Here's how the part is built. I have some questions about the finished solid (model axes, mm). A direction names the side the tool comes from. Give positions to 0.01 mm unless a question says otherwise; leave off trailing zeros. Write each loop counter-clockwise with the first axis right and the second up, starting at its lowest first coordinate (ties: lowest second). Pieces come first, ordered by that corner, then holes. Notation, with made-up numbers: (55, 51) -> (73, 51) arc R33 cw to (73, 82) -> close; hole circle Ø7 at (-17.75, 19). An arc over 180 degrees is marked (long way). Return JSON: item names as keys, results as strings.
from build123d import *

# Parameters (mm, degrees)
HOLE_WIZARD_M8_1_D           = 6.8
HOLE_WIZARD_M8_1_CSINK_D     = 8.05
HOLE_WIZARD_M8_1_CSINK_ANGLE = 90


with BuildPart() as part:
    # 草图1 → 旋转1 (revolve)
    with BuildSketch(Plane.XY, mode=Mode.PRIVATE) as revolve_1_sk:
        Polygon((0, 0), (77.5, 0), (77.5, 8), (45, 8), (45, 21), (37.5, 21), (37.5, 8), (0, 8), align=None)
    revolve(revolve_1_sk.sketch.rotate(Axis((0, 8, 0), (0, -1, 0)), 180), axis=Axis((0, 8, 0), (0, -1, 0)))

    # M8 螺纹孔1 (through all)
    with Locations(Plane(origin=(0, 8, 0), x_dir=(1, 0, 0), z_dir=(0, 1, 0))):
        with Locations((-67.5, 0), (67.5, 0), (0, -67.5), (0, 67.5)):
            CounterSinkHole(HOLE_WIZARD_M8_1_D / 2, HOLE_WIZARD_M8_1_CSINK_D / 2, counter_sink_angle=HOLE_WIZARD_M8_1_CSINK_ANGLE)


solid = part.part
1. Suppose I cut it at D-D, the plane x = 16. List the corners of the cut face in (y, z) for me, and give its area (3 significant figures).
Taken from the geometry:
{"outline": "(0, -75.83) -> (8, -75.83) -> (8, -42.06) -> (21, -42.06) -> (21, -33.92) -> (8, -33.92) -> (8, 33.92) -> (21, 33.92) -> (21, 42.06) -> (8, 42.06) -> (8, 75.83) -> (0, 75.83) -> close", "area": "1,430 mm²"}
2. Which directions (+Z, -Z, +X, -X, +Y, -Y) give clear straight access to the entire face, cutting with the end or side of a thin tool? Please do faces 1 (the face through (1, 8, -1)), 2 (the face through (17, 21, -34)).
Taken from the geometry:
{"face 1": "+Y", "face 2": "+Z, -Z, +X, -X, +Y"}
3. If I drill on line 1 (Z direction, x = 0, y = 4); line 2 (Y direction, x = -69, z = -4.5); line 3 (X direction, y = 4.5, z = 67.5), over which ranges is the centre line in solid material (lowest first)? Write a range as [from, to].
Taken from the geometry:
{"line 1": "z = [-77.5, -70.9], [-64.1, 64.1], [70.9, 77.5]", "line 2": "y = [0, 8]", "line 3": "x = [-38.08, -3.4], [3.4, 38.08]"}
4. For pin 1 Ø10 at (x, y) = (57, 2.5) entering from +Z; pin 2 Ø9 at (x, z) = (0, 67.5) entering from -Y; pin 3 Ø5 at (y, z) = (7, -56) entering from -X; pin 4 Ø1.5 at (x, y) = (3, 16) entering from -Z, each with a flat end and sliding along its axis, tell me the tip position at first contact or that it passes through.
Taken from the geometry:
{"pin 1": "stops at z = 57.47", "pin 2": "stops at y = 0", "pin 3": "stops at x = -56.07", "pin 4": "stops at z = -44.94"}
5. Suppose I cut it at C-C, the plane z = -67.5. List the corners of the cut face in (x, y) for me (3 decimals), and give its area (3 significant figures).
Taken from the geometry:
{"outline": "(-38.079, 0) -> (-3.4, 0) -> (-3.4, 7.375) -> (-4.025, 8) -> (-38.079, 8) -> close; (3.4, 0) -> (38.079, 0) -> (38.079, 8) -> (4.025, 8) -> (3.4, 7.375) -> close", "area": "554 mm²"}
6. Suppose I cut it at A-A, the plane z = 0. List the corners of the cut face in (x, y) for me (3 decimals), and give its area (3 significant figures).
Taken from the geometry:
{"outline": "(-77.5, 0) -> (-70.9, 0) -> (-70.9, 7.375) -> (-71.525, 8) -> (-77.5, 8) -> close; (-64.1, 0) -> (64.1, 0) -> (64.1, 7.375) -> (63.475, 8) -> (45, 8) -> (45, 21) -> (37.5, 21) -> (37.5, 8) -> (-37.5, 8) -> (-37.5, 21) -> (-45, 21) -> (-45, 8) -> (-63.475, 8) -> (-64.1, 7.375) -> close; (70.9, 0) -> (77.5, 0) -> (77.5, 8) -> (71.525, 8) -> (70.9, 7.375) -> close", "area": "1,330 mm²"}
7. Suppose I cut it at B-B, the plane x = 0. List the corners of the cut face in (y, z) for me (3 decimals).
Taken from the geometry:
{"outline": "(0, -77.5) -> (8, -77.5) -> (8, -71.525) -> (7.375, -70.9) -> (0, -70.9) -> close; (0, -64.1) -> (7.375, -64.1) -> (8, -63.475) -> (8, -45) -> (21, -45) -> (21, -37.5) -> (8, -37.5) -> (8, 37.5) -> (21, 37.5) -> (21, 45) -> (8, 45) -> (8, 63.475) -> (7.375, 64.1) -> (0, 64.1) -> close; (0, 70.9) -> (7.375, 70.9) -> (8, 71.525) -> (8, 77.5) -> (0, 77.5) -> close"}
8. If we mould it in two halves opening along Z, with no side actions, what happens to faces 3 (the face through (-33, 8, 33)), 4 (the face through (-35.762, 4.056, 68.756)), 5 (the face through (0.74, 3.64, 70.82)), 6 (the face through (64.257, 3.636, -1.021))? For each: released by +Z, released by -Z, zero draft, split by the parting line, or undercut.
Taken from the geometry:
{"face 3": "zero draft", "face 4": "split by the parting line", "face 5": "undercut", "face 6": "undercut"}
